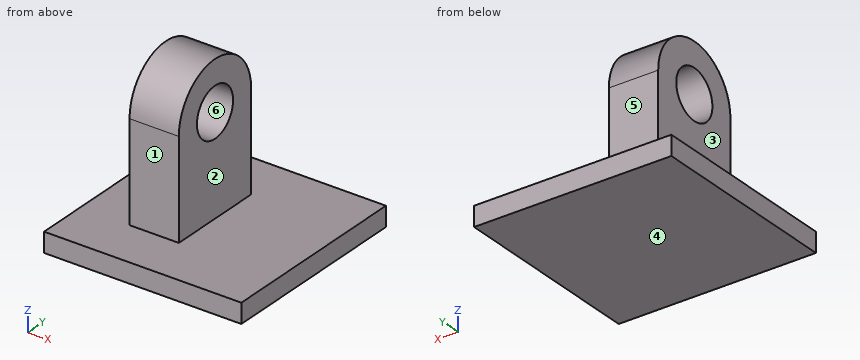
from build123d import *

# Parameters (mm, degrees)
F0_W     = 254
F0_H     = 254
F1_DEPTH = 25.4
F2_W     = 63.5
F2_H     = 127
F3_DEPTH = 127
F4_R     = 63.5
F5_DEPTH = 63.5
F6_R     = 31.75
F7_DEPTH = 63.5


with BuildPart() as f1:
    # F0 (on Top) → F1 (new body)
    with BuildSketch(Plane.XY):
        Rectangle(F0_W, F0_H)
    extrude(amount=F1_DEPTH)

    # F2 (on face) → F3 (join)
    with BuildSketch(Plane.XY.offset(25.4)):
        with Locations((-31.75, 0)):
            Rectangle(F2_W, F2_H)
    extrude(amount=F3_DEPTH)

    # F4 (on face) → F5 (join)
    with BuildSketch(Plane(origin=(-63.5, 0, 0), x_dir=(0, -1, 0), z_dir=(-1, 0, 0))):
        with Locations((0, 152.4)):
            Circle(F4_R)
    extrude(amount=-F5_DEPTH)

    # F6 (on face) → F7 (cut, through all)
    with BuildSketch(Plane.YZ):
        with Locations((0, 152.4)):
            Circle(F6_R)
    extrude(amount=-F7_DEPTH, mode=Mode.SUBTRACT)


solid = f1.part
Geometry check sheet. Reference: the model listing, model coordinates, mm. Face numbers are marked on the shaded views. A direction names the side the tool comes from. Round coordinates to 2 decimals unless told otherwise and drop trailing zeros. Write each loop counter-clockwise with the first axis right and the second up, starting at its lowest first coordinate (ties: lowest second). Pieces come first, ordered by that corner, then holes. Notation, with made-up numbers: (-26, 11) - (-20, 11) arc R29 ccw to (-20, 48) - close; hole circle Ø5 at (71.5, 75). An arc over 180 degrees is marked (long way). One line per item, written item: value.
1. Set-up check for the marked faces 1, 2 and 3: record each of +Z, -Z, +X, -X, +Y, -Y from which the full face is reachable in a straight line by a thin tool's end or side.
The answers:
face 1: +Z, +X, -X, -Y
face 2: +Z, +X, +Y, -Y
face 3: +Z, -X, +Y, -Y
2. Cross-section at C-C on z = 126. Record the boundary of the cut face in (x, y), and give its area (3 significant figures).
The answers:
outline: (-63.5, -63.5) - (0, -63.5) - (0, -17.64) - (-63.5, -17.64) - close; (-63.5, 17.64) - (0, 17.64) - (0, 63.5) - (-63.5, 63.5) - close
area: 5,820 mm^2
3. Scan lines: L1, parallel to Z at x = -25.5, y = 0; L2, parallel to Z at x = 69, y = -81; L3, parallel to Y at x = -51, z = 152. Record each from-to range of solid material in increasing order.
The answers:
L1: z = 0 to 120.65, 184.15 to 215.9
L2: z = 0 to 25.4
L3: y = -63.5 to -31.75, 31.75 to 63.5
4. Depth check by flat-ended pin: pin 1 Ø10 at (y, z) = (-62, 164) entering from +X; pin 2 Ø5 at (x, z) = (-47.5, 62.5) entering from -Y; pin 3 Ø1.5 at (x, y) = (86.5, 88.5) entering from +Z. Enter the tip coordinate at first touch or a pass-through.
The answers:
pin 1: stops at x = 0
pin 2: stops at y = -63.5
pin 3: stops at z = 25.4
5. Cross-section at D-D on y = 88. Record the boundary of the cut face in (x, z).
The answers:
outline: (-127, 0) - (127, 0) - (127, 25.4) - (-127, 25.4) - close
6. Mould release check, pull along Z, two halves, no side actions. Record for the marked faces 4, 5 and 6: released by +Z, released by -Z, zero draft, split by the parting line, or undercut.
The answers:
face 4: released by -Z
face 5: zero draft
face 6: undercut
7. Cross-section at A-A on y = 0. Record the boundary of the cut face in (x, z).
The answers:
outline: (-127, 0) - (127, 0) - (127, 25.4) - (0, 25.4) - (0, 120.65) - (-63.5, 120.65) - (-63.5, 25.4) - (-127, 25.4) - close; (-63.5, 184.15) - (0, 184.15) - (0, 215.9) - (-63.5, 215.9) - close
8. Cross-section at B-B on x = -59. Record the boundary of the cut face in (y, z), and give its area (3 significant figures).
The answers:
outline: (-127, 0) - (127, 0) - (127, 25.4) - (63.5, 25.4) - (63.5, 152.4) arc R63.5 ccw to (-63.5, 152.4) - (-63.5, 25.4) - (-127, 25.4) - close; hole circle Ø63.5 at (0, 152.4)
area: 25,700 mm^2
